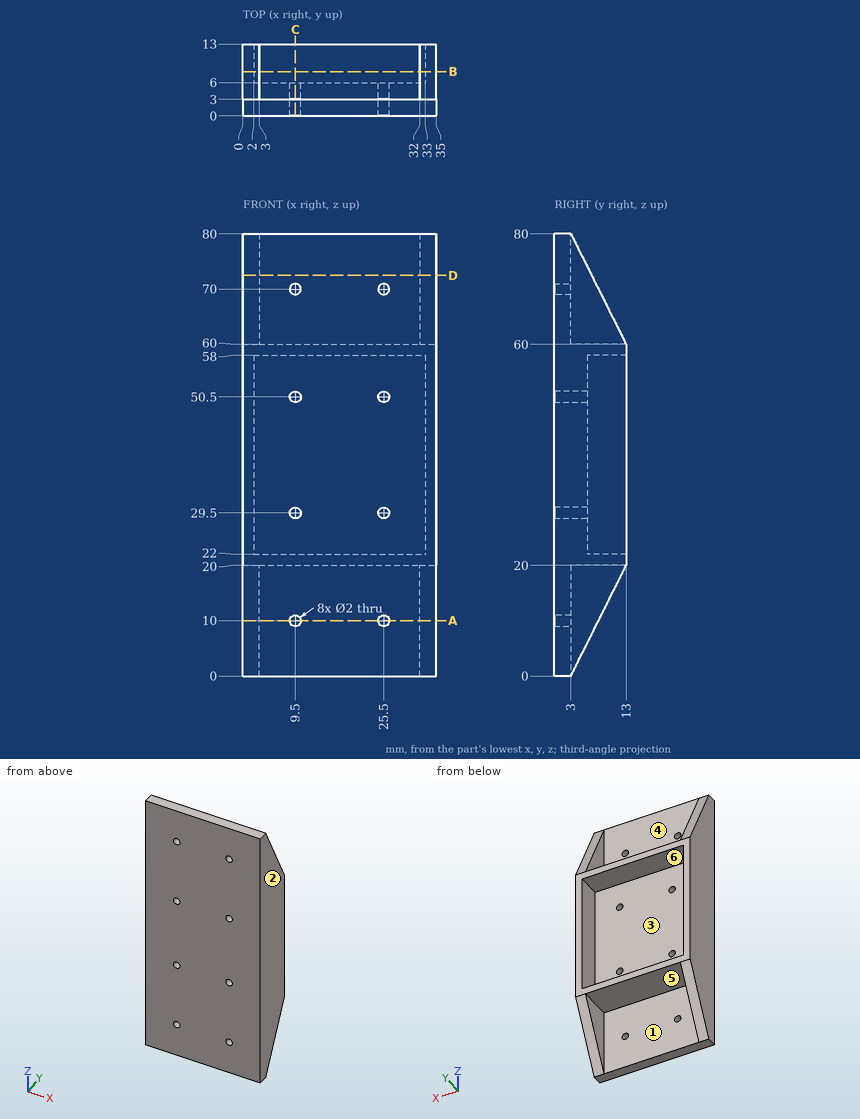
Check sheet for the drawn part. Datum: minimum x, y, z corner. Units: mm. A direction names the side the tool comes from. Round coordinates to 2 decimals unless told otherwise and drop trailing zeros. Loops run counter-clockwise (first coordinate to the right, second up) from the corner with the lowest first, then second, coordinate; pieces in that order, holes last. Notation, with made-up numbers: (47.25, 50) - (52.25, 50) arc R8 cw to (52.25, 60) - close; hole circle Ø11 at (39.25, -26). An arc over 180 degrees is marked (long way). Write item = value, one per line. Start each with the question number.
1. Section check D-D on z = 72.5. Enter the section's corners in (x, y), then the cut area to 4 significant figures.
2. Thickness scan on line 1 (X direction, y = 1.45, z = 70); line 2 (X direction, y = 9.5, z = 17); line 3 (Z direction, x = 12, y = 7.75). Record the ranges inside material, lowest first.
3. Mould release check, pull along Z, two halves, no side actions. Record for the marked faces 4, 5 and 6: released by +Z, released by -Z, zero draft, split by the parting line, or undercut.
4. Section check B-B on y = 8. Enter the section's corners in (x, z).
5. Depth check by flat-ended pin: pin 1 (4 mm diameter, centred on x = 16, y = 9.5, fed in from -Z); pin 2 (2 mm diameter, centred on x = 22, z = 52.5, fed in from +Y); pin 3 (5 mm diameter, centred on y = 3.5, z = 42, fed in from -X); pin 4 (3 mm diameter, centred on x = 14, y = 7.5, fed in from +Z). Enter the tip coordinate at first touch or a pass-through.
6. Section check A-A on z = 10. Enter the section's corners in (x, y), then the cut area to 3 significant figures.
7. Section check C-C on x = 9.5. Enter the section's corners in (y, z).
8. Set-up check for the marked faces 1, 2 and 3: record each of +Z, -Z, +X, -X, +Y, -Y from which the full face is reachable in a straight line by a thin tool's end or side.
Working result:
q1.outline = (0, 0) - (35, 0) - (35, 6.75) - (32, 6.75) - (32, 3) - (3, 3) - (3, 6.75) - (0, 6.75) - close
q1.area = 127.5 mm^2
q2.line_1 = 0 to 8.5, 10.5 to 24.5, 26.5 to 35
q2.line_2 = 0 to 3, 32 to 35
q2.line_3 = 20 to 22, 58 to 60
q3.face_4 = zero draft
q3.face_5 = released by -Z
q3.face_6 = undercut
q4.outline = (0, 10) - (3, 10) - (3, 20) - (32, 20) - (32, 10) - (35, 10) - (35, 70) - (32, 70) - (32, 60) - (3, 60) - (3, 70) - (0, 70) - close; hole (2, 22) - (33, 22) - (33, 58) - (2, 58) - close
q5.pin_1 = 20
q5.pin_2 = 6
q5.pin_3 = 0
q5.pin_4 = 60
q6.outline = (0, 0) - (8.5, 0) - (8.5, 3) - (3, 3) - (3, 8) - (0, 8) - close; (10.5, 0) - (24.5, 0) - (24.5, 3) - (10.5, 3) - close; (26.5, 0) - (35, 0) - (35, 8) - (32, 8) - (32, 3) - (26.5, 3) - close
q6.area = 123 mm^2
q7.outline = (0, 0) - (3, 0) - (3, 9) - (0, 9) - close; (0, 11) - (3, 11) - (3, 20) - (13, 20) - (13, 22) - (6, 22) - (6, 28.5) - (0, 28.5) - close; (0, 30.5) - (6, 30.5) - (6, 49.5) - (0, 49.5) - close; (0, 51.5) - (6, 51.5) - (6, 58) - (13, 58) - (13, 60) - (3, 60) - (3, 69) - (0, 69) - close; (0, 71) - (3, 71) - (3, 80) - (0, 80) - close
q8.face_1 = -Z, +Y
q8.face_2 = +Z, -Z, +X, +Y, -Y
q8.face_3 = +Y
